Build history of the part. All positions in model axes, mm. A direction names the side the tool comes from. Give positions to 0.01 mm unless a question says otherwise; leave off trailing zeros. Order: outer loops, then holes, each group sorted by start corner. A loop starts at its lowest first (then second) coordinate and runs counter-clockwise, first axis right, second up. Notation, with made-up numbers: (69.5, -39) -> (114.5, -39) arc R19 ccw to (114.5, -22) -> close; hole circle Ø7 at (-23.5, 21). An arc over 180 degrees is marked (long way). One line per item, written item: value. Start each with the question number.
(1) Saw through at A-A on x = 0. Give the cut face in (y, z), plus the area to 3 significant figures.
(2) Saw through at C-C on z = -12.5. Give the cut face in (x, y), plus the area to 3 significant figures.
(3) Saw through at B-B on y = -48.5. Give the cut face in (x, z).
(4) Which spindle directions (+Z, -Z, +X, -X, +Y, -Y) get a long thin tool onto all of the face, cutting with end or side? Do faces 1 (the flat face through (-0.3, 2.3, -14)), 2 (the flat face through (4, -25, -25)), 3 (the flat face through (0, 2, -7)), 4 (the cylindrical face through (0.521, -53.966, -50.101)). Say none if no direction does.
(5) Pin check, flat tips, straight feed: pin 1 (4 mm diameter, centred on x = 0, y = -26.5, fed in from -Z); pin 2 (2 mm diameter, centred on x = -1, y = -1, fed in from +Z); pin 3 (1.3 mm diameter, centred on x = 0, z = -8, fed in from +Y); pin 4 (4 mm diameter, centred on x = 0.5, y = -20.5, fed in from +Z). Stop position of each tip, or through.
(6) Probe line 1 (Z direction, x = 0.5, y = -14); line 2 (Z direction, x = -1.25, y = -50); line 3 (Y direction, x = -1.75, z = -39). List the from-to ranges inside material, lowest first.
(7) Saw through at D-D on z = -38. Give the cut face in (x, y).
Autodesk Inventor part; units mm, degrees
ref_plane "YZ Plane" through (0, 0, 0) normal (1, 0, 0) x (0, 1, 0)
ref_plane "XZ Plane" through (0, 0, 0) normal (0, 1, 0) x (-1, 0, 0)
ref_plane "XY Plane" through (0, 0, 0) normal (0, 0, 1) x (1, 0, 0)
sketch "Sketch1" plane through (0, 0, 0) normal (1, 0, 0) x (0, 1, 0)
  line L0 (0, 0) -> (2.9, 0)
  line L1 (2.9, 0) -> (2.9, -14)
  line L2 (0, -14) -> (0, 0)
  line L3 (2.9, -14) -> (3.5, -14)
  line L4 (3.5, -14) -> (3.5, -22)
  line L5 (3.5, -22) -> (0, -22)
  line L6 (0, -22) -> (0, -14)
  dimension "d0" = 14
  dimension "d1" = 3.5
  dimension "d2" = 8
  dimension "d3" = 2.9
revolve "Revolution1" add sketch "Sketch1" angle 360 about axis through (0, 0, -22) along (0, 0, 1)
sketch "Sketch2" plane through (0, 0, -22) normal (0, 0, -1) x (-1, 0, 0)
  circle A0 centre (0, 0) radius 4
  line L0 (-4, 0) -> (4, 0)
  line L1 (4, 0) -> (4, -50)
  line L2 (4, -50) -> (-4, -50)
  line L3 (-4, -50) -> (-4, 0)
  circle A1 centre (0, -50) radius 4
  point P0 (4, 0)
  dimension "d5" = 8
  dimension "d6" = 50
extrude "Extrusion1" add sketch "Sketch2" along normal blind 7
sketch "Sketch3" plane through (0, 0, -29) normal (0, 0, -1) x (-1, 0, 0)
  arc A0 (-4, -50) -> (4, -50) centre (0, -50) ccw
  circle A1 centre (0, -50) radius 4
  point P0 (0, 0)
  point P1 (4, -50)
  point P2 (-4, -50)
extrude "Extrusion2" add sketch "Sketch3" along normal blind 50
sketch "Sketch4" plane through (0, 0, 0) normal (0, 0, 1) x (1, 0, 0)
  line L0 (2.1, 2) -> (-2.1, 2)
  arc A0 (2.1, 2) -> (-2.1, 2) centre (0, 0) ccw
  dimension "d11" = 2
extrude "Extrusion3" cut sketch "Sketch4" against normal up to surface (14 mm away)
properties part number "HandCrank"
Results below:
1. outline: (-54, -79) -> (-46, -79) -> (-46, -29) -> (4, -29) -> (4, -22) -> (3.5, -22) -> (3.5, -14) -> (2, -14) -> (2, 0) -> (-2.9, 0) -> (-2.9, -14) -> (-3.5, -14) -> (-3.5, -22) -> (-54, -22) -> close
1. area: 931 mm²
2. outline: (-2.1, 2) arc R2.9 ccw (long way) to (2.1, 2) -> close
2. area: 23.8 mm²
3. outline: (-4, -29) -> (-3.71, -29) -> (-3.71, -79) -> (3.71, -79) -> (3.71, -29) -> (4, -29) -> (4, -22) -> (-4, -22) -> close
4. face 1: +Z
4. face 2: +Z, -Z, +X, +Y, -Y
4. face 3: +Z, +X, -X, +Y
4. face 4: -Z
5. pin 1: stops at z = -29
5. pin 2: stops at z = 0
5. pin 3: stops at y = 2
5. pin 4: stops at z = -22
6. line 1: z = -29 to -22
6. line 2: z = -79 to -22
6. line 3: y = -53.6 to -46.4
7. outline: circle Ø8 at (0, -50)
